```python
from build123d import *

# Parameters (mm, degrees)
SKETCH_1_W          = 24
SKETCH_1_H          = 28
EXTRUDE_1_DEPTH     = 6
SKETCH_2_W          = 17.5
SKETCH_2_H          = 18.5
CUT_EXTRUDE_3_DEPTH = 5
SKETCH_4_R          = 1
CUT_EXTRUDE_4_DEPTH = 5
SKETCH_5_W          = 3.75
SKETCH_5_H          = 18.5
CUT_EXTRUDE_5_DEPTH = 5
FILLET_1_R          = 3
SKETCH_7_R          = 1.5
EXTRUDE_4_DEPTH     = 6
SKETCH_12_R         = 1.5
CUT_EXTRUDE_6_DEPTH = 10


with BuildPart() as part:
    # 草图1 → 凸台-拉伸1 (new body)
    with BuildSketch(Plane(origin=(0, 0, 0), x_dir=(1, 0, 0), z_dir=(0, 1, 0))):
        with Locations((12, -14)):
            Rectangle(SKETCH_1_W, SKETCH_1_H)
    extrude(amount=EXTRUDE_1_DEPTH)

    # 草图2 → 切除-拉伸3 (cut)
    with BuildSketch(Plane(origin=(0, 6, 0), x_dir=(1, 0, 0), z_dir=(0, 1, 0))):
        with Locations((11.5, -14)):
            Rectangle(SKETCH_2_W, SKETCH_2_H)
    extrude(amount=-CUT_EXTRUDE_3_DEPTH, mode=Mode.SUBTRACT)

    # 草图4 → 切除-拉伸4 (cut)
    with BuildSketch(Plane(origin=(0, 1, 0), x_dir=(1, 0, 0), z_dir=(0, 1, 0))):
        with Locations(Location((6, -7, 0), (0, 0, 270))):
            Circle(SKETCH_4_R)
        with Locations(Location((17, -7, 0), (0, 0, 270))):
            Circle(SKETCH_4_R)
        with Locations(Location((6, -21, 0), (0, 0, 270))):
            Circle(SKETCH_4_R)
        with Locations(Location((17, -21, 0), (0, 0, 270))):
            Circle(SKETCH_4_R)
        with BuildLine():
            Line((8.95, -10.25), (14.05, -10.25))
            ThreePointArc((14.05, -10.25), (17.8, -14), (14.05, -17.75))
            Line((14.05, -17.75), (8.95, -17.75))
            ThreePointArc((8.95, -17.75), (5.2, -14), (8.95, -10.25))
        make_face()
    extrude(amount=-CUT_EXTRUDE_4_DEPTH, mode=Mode.SUBTRACT)

    # 草图5 → 切除-拉伸5 (cut)
    with BuildSketch(Plane(origin=(0, 6, 0), x_dir=(1, 0, 0), z_dir=(0, 1, 0))):
        with Locations((22.125, -14)):
            Rectangle(SKETCH_5_W, SKETCH_5_H)
    extrude(amount=-CUT_EXTRUDE_5_DEPTH, mode=Mode.SUBTRACT)

    # 圆角1
    fillet_1_edges = [part.edges().sort_by_distance(p)[0] for p in [
        (0, 3, 0),
        (0, 3, 28),
    ]]
    fillet(fillet_1_edges, radius=FILLET_1_R)

    # 草图7 → 凸台-拉伸4 (add)
    # profile 1 of 2: a face of its own
    with BuildSketch(Plane(origin=(0, 6, 0), x_dir=(1, 0, 0), z_dir=(0, 1, 0))):
        with BuildLine():
            Line((12.846291202, 0), (10.153708798, 0))
            ThreePointArc((10.153708798, 0), (11.5, -7.25), (12.846291202, 0))
        make_face()
        with Locations((11.5, -3.5)):
            Circle(SKETCH_7_R, mode=Mode.SUBTRACT)
    # profile 2 of 2: a face of its own
    with BuildSketch(Plane(origin=(0, 6, 0), x_dir=(1, 0, 0), z_dir=(0, 1, 0))):
        with BuildLine():
            Line((12.846291202, -28), (10.153708798, -28))
            ThreePointArc((10.153708798, -28), (11.5, -20.75), (12.846291202, -28))
        make_face()
        with Locations((11.5, -24.5)):
            Circle(SKETCH_7_R, mode=Mode.SUBTRACT)
    extrude(amount=-EXTRUDE_4_DEPTH)

    # 草图12 → 切除-拉伸6 (cut)
    with BuildSketch(Plane(origin=(0, 6, 0), x_dir=(1, 0, 0), z_dir=(0, 1, 0))):
        with Locations(Location((11.5, -3.5, 0), (0, 0, 270))):
            Circle(SKETCH_12_R)
        with Locations(Location((11.5, -24.5, 0), (0, 0, 270))):
            Circle(SKETCH_12_R)
    extrude(amount=-CUT_EXTRUDE_6_DEPTH, mode=Mode.SUBTRACT)


solid = part.part
```
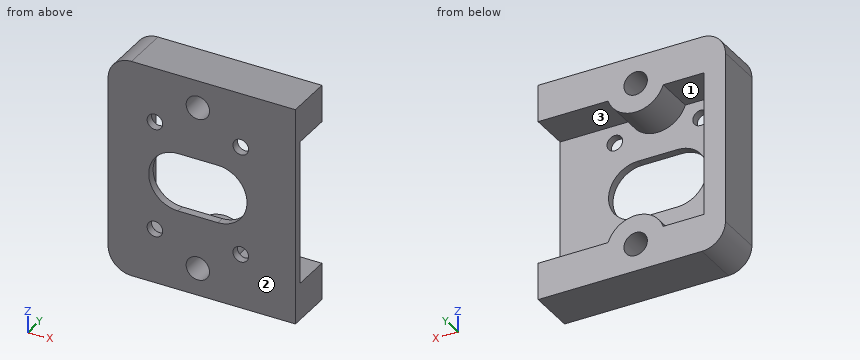
For this review, take the finished solid that the model builds, in its own axes (mm). Face numbers are marked on the shaded views. A direction names the side the tool comes from. Round coordinates to 2 decimals unless told otherwise and drop trailing zeros. Write each loop counter-clockwise with the first axis right and the second up, starting at its lowest first coordinate (ties: lowest second). Pieces come first, ordered by that corner, then holes. Notation, with made-up numbers: (6, -23.5) - (24, -23.5) arc R31 cw to (24, 5.5) - close; hole circle Ø4 at (48, -5). An arc over 180 degrees is marked (long way). Write each question's results on one line, items separated by ' | '.
Item 1: Take a section at C-C on x = 6. State the section outline as (y, z) points, then the cut area to 3 significant figures.
Calculated:
outline: (0, 0) - (6, 0) - (6, 4.75) - (1, 4.75) - (1, 6) - (0, 6) - close; (0, 8) - (1, 8) - (1, 11.68) - (0, 11.68) - close; (0, 16.32) - (1, 16.32) - (1, 20) - (0, 20) - close; (0, 22) - (1, 22) - (1, 23.25) - (6, 23.25) - (6, 28) - (0, 28) - close | area: 66.9 mm^2
Item 2: For the marked faces 1, 2 and 3, list the 3-axis set-ups (+Z, -Z, +X, -X, +Y, -Y) from which the entire face can be reached by the end or side of a thin tool; tool diameter is ignored.
Calculated:
face 1: +Y | face 2: +Z, -Z, +X, -X, -Y | face 3: +X, +Y
Item 3: Take a section at A-A on x = 9.25. State the section outline as (y, z) points, then the cut area to 3 significant figures.
Calculated:
outline: (0, 0) - (6, 0) - (6, 6.5) - (1, 6.5) - (1, 10.25) - (0, 10.25) - close; (0, 17.75) - (1, 17.75) - (1, 21.5) - (6, 21.5) - (6, 28) - (0, 28) - close | area: 85.5 mm^2
Item 4: Take a section at D-D on z = 11. State the section outline as (x, y) points.
Calculated:
outline: (0, 0) - (6.7, 0) - (6.7, 1) - (2.75, 1) - (2.75, 6) - (0, 6) - close; (16.3, 0) - (24, 0) - (24, 1) - (16.3, 1) - close
Item 5: Take a section at B-B on z = 24.5. State the section outline as (x, y) points, then the cut area to 3 significant figures.
Calculated:
outline: (0, 0) - (10, 0) - (10, 6) - (0, 6) - close; (13, 0) - (24, 0) - (24, 6) - (13, 6) - close | area: 126 mm^2
Item 6: To check wall thickness, follow line 1 along X through (y, z) = (0.35, 21); line 2 along Z through (x, y) = (23.25, 2.4); line 3 along X through (y, z) = (1.5, 24.5). State the ranges of each line that lie inside material, in increasing order. Write a range as from..to.
Calculated:
line 1: x = 0..5, 7..16, 18..24 | line 2: z = 0..4.75, 23.25..28 | line 3: x = 0..10, 13..24
Item 7: For pin 1 (5.5 mm diameter, centred on x = 9, z = 10.5, fed in from +Y); pin 2 (1.6 mm diameter, centred on x = 6, z = 7, fed in from -Y); pin 3 (2.5 mm diameter, centred on y = 3, z = 11.5, fed in from +X); pin 4 (1.5 mm diameter, centred on y = 2.5, z = 20.5, fed in from +X), all flat-tipped, find the tip position at first contact; note any pin that passes through.
Calculated:
pin 1: stops at y = 1 | pin 2: passes through | pin 3: stops at x = 2.75 | pin 4: stops at x = 13.37
